Autodesk Inventor part; units mm, degrees
ref_plane "YZ Plane" through (0, 0, 0) normal (1, 0, 0) x (0, 1, 0)
ref_plane "XZ Plane" through (0, 0, 0) normal (0, 1, 0) x (-1, 0, 0)
ref_plane "XY Plane" through (0, 0, 0) normal (0, 0, 1) x (1, 0, 0)
sketch "Эскиз1" plane through (0, 0, 0) normal (0, 0, 1) x (1, 0, 0)
  line L0 (0, 0) -> (140, 0)
  line L1 (140, 0) -> (140, 140)
  line L2 (140, 140) -> (0, 140)
  line L3 (0, 140) -> (0, 0)
  circle A0 centre (70, 70) radius 50
  line L4 (0, 140) -> (20, 140)
  line L5 (20, 140) -> (20, 120)
  line L6 (140, 0) -> (140, 20)
  line L7 (140, 20) -> (120, 20)
  line L8 (20, 120) -> (120, 120)
  line L9 (120, 120) -> (120, 20)
  line L10 (120, 20) -> (20, 20)
  line L11 (20, 20) -> (20, 120)
  line L12 (70, 70) -> (0, 70)
  line L13 (0, 70) -> (0, 0)
  line L14 (0, 0) -> (70, 0)
  line L15 (70, 0) -> (70, 70)
  circle A1 centre (20, 120) radius 3
  circle A2 centre (120, 120) radius 3
  circle A3 centre (120, 20) radius 3
  circle A4 centre (20, 20) radius 3
  dimension "d0" = 140
  dimension "d1" = 140
  dimension "d2" = 100
  dimension "d3" = 20
  dimension "d4" = 20
  dimension "d5" = 20
  dimension "d6" = 20
  dimension "d7" = 70
  dimension "d8" = 70
  dimension "d9" = 6
  dimension "d10" = 6
  dimension "d11" = 6
  dimension "d14" = 6
extrude "Выдавливание1" add sketch "Эскиз1" along normal blind 4 contours L3 L12 L11 A4 L10 L15 L0 | L15 L10 A3 L7 L1 L0 | L3 L2 L5 A1 L11 L12 | L10 A4 L11 A0 | A0 L9 A3 L10 | L11 A1 L8 A0 | L7 A3 L9 A2 L8 A1 L5 L2 L1 | A0 L8 A2 L9
sketch "Эскиз2" plane through (0, 140, 0) normal (0, 1, 0) x (1, 0, 0)
  line L0 (0, 0) -> (0, -4)
  line L1 (0, 0) -> (140, 0)
  line L2 (140, 0) -> (140, -50)
  line L3 (140, -50) -> (0, -50)
  line L4 (0, -50) -> (0, 0)
  line L5 (0, -25) -> (20, -25)
  line L6 (140, -25) -> (120, -25)
  circle A0 centre (120, -25) radius 3
  circle A1 centre (20, -25) radius 3
  line L7 (140, 0) -> (0, 0)
  line L8 (0, 0) -> (0, 50)
  line L9 (0, 50) -> (140, 50)
  line L10 (140, 50) -> (140, 0)
  line L11 (140, 25) -> (120, 25)
  circle A2 centre (120, 25) radius 3
  circle A3 centre (20, 25) radius 3
  line L12 (0, 25) -> (20, 25)
  point P0 (0, -4)
  point P1 (0, 0)
  dimension "d15" = 140
  dimension "d16" = 50
  dimension "d17" = 20
  dimension "d18" = 20
  dimension "d19" = 6
  dimension "d20" = 6
  dimension "d23" = 140
  dimension "d24" = 50
  dimension "d25" = 6
  dimension "d26" = 6
  dimension "d30" = 20
extrude "Выдавливание2" add sketch "Эскиз2" along normal blind 8
sketch "Эскиз3" plane through (0, 0, 0) normal (0, 0, -1) x (-1, 0, 0)
  line L0 (0, 0) -> (-140, 0)
  line L1 (-140, 140) -> (0, 140)
  line L2 (-140, 0) -> (0, 0)
  line L3 (0, 0) -> (0, 140)
  line L4 (0, 140) -> (-140, 140)
  line L5 (-140, 140) -> (-140, 0)
  circle A0 centre (-120, 20) radius 3
  circle A1 centre (-120, 120) radius 3
  circle A2 centre (-20, 120) radius 3
  circle A3 centre (-20, 20) radius 3
  circle A4 centre (-70, 70) radius 35
  circle A5 centre (-70, 70) radius 50
  dimension "d27" = 70
extrude "Выдавливание3" add sketch "Эскиз3" along normal blind 4 contours L0 L5 L1 L3 | A5
chamfer "Фаска1" distance 1 angle 45 19 edges at (23, 20, -4) (105, 70, -4) (123, 20, -4) (123, 120, -4) (117, 140, -25) (17, 140, -25) (23, 120, -4) (20, 70, 4) (105, 70, 0) (117, 120, 4) (117, 140, 25) (17, 140, 25) (17, 120, 4) (17, 20, 4) (117, 20, 4) (17, 148, 25) (17, 148, -25) (117, 148, 25) (117, 148, -25)
properties part number "Кронштейн мотора"
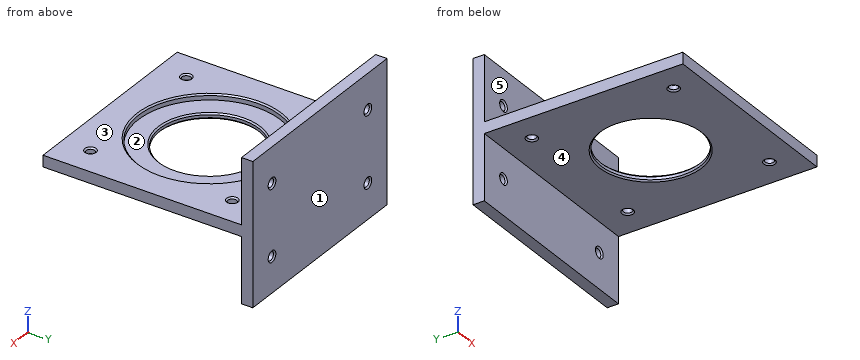
The listing builds one solid part. Answer for the finished solid, in the listing's coordinates (mm). Face numbers are marked on the shaded views. A direction names the side the tool comes from. Round coordinates to 2 decimals unless told otherwise and drop trailing zeros. Loops run counter-clockwise (first coordinate to the right, second up) from the corner with the lowest first, then second, coordinate; pieces in that order, holes last.
Q1. Given pin 1 Ø8 at (x, y) = (46, 18) entering from +Z; pin 2 Ø7 at (x, y) = (120, 20) entering from -Z; pin 3 Ø5 at (x, y) = (22, 131.5) entering from -Z, each flat-ended and moving along its own axis, determine where each tip first touches the part or whether it passes through.
Q2. Section A-A, the plane y = 70 is taken. Determine the outline of the cut face in (x, z).
Q3. Section B-B, the plane x = 70 is taken. Determine the outline of the cut face in (y, z), then the cut area to 3 significant figures.
Q4. Find the intervals of material crossed by line 1 (Z direction, x = 120, y = 144.4); line 2 (Y direction, x = 120, z = -0.7); line 3 (X direction, y = 20, z = -1.2), in increasing order.
Q5. Which of the six approach directions +Z, -Z, +X, -X, +Y, -Y give full straight-line access (tool end or side, diameter ignored) to the marked faces 4 and 5?
Q6. Section C-C, the plane z = 13 is taken. Determine the outline of the cut face in (x, y).
Q7. For a pull along Y with two mould halves and no side action, classify the marked faces 1, 2 and 3 as released by +Y, released by -Y, zero draft, split by the parting line, or undercut.
Completed:
1. pin 1: stops at z = 4
1. pin 2: stops at z = -3.5
1. pin 3: stops at z = -4
2. outline: (0, -4) - (34, -4) - (35, -3) - (35, -1) - (34, 0) - (20, 0) - (20, 3) - (19, 4) - (0, 4) - close; (105, -3) - (106, -4) - (140, -4) - (140, 4) - (121, 4) - (120, 3) - (120, 0) - (106, 0) - (105, -1) - close
3. outline: (0, -4) - (34, -4) - (35, -3) - (35, -1) - (34, 0) - (20, 0) - (20, 3) - (19, 4) - (0, 4) - close; (105, -3) - (106, -4) - (140, -4) - (140, -50) - (148, -50) - (148, 50) - (140, 50) - (140, 4) - (121, 4) - (120, 3) - (120, 0) - (106, 0) - (105, -1) - close
3. area: 1,240 mm2
4. line 1: z = -50 to -28, -22 to 22, 28 to 50
4. line 2: y = 0 to 17, 23 to 117, 123 to 148
4. line 3: x = 0 to 17, 23 to 117, 123 to 140
5. face 4: -Z, +X, -X, -Y
5. face 5: +Z, +X, -X, -Y
6. outline: (0, 140) - (140, 140) - (140, 148) - (0, 148) - close
7. face 1: released by +Y
7. face 2: undercut
7. face 3: zero draft
